Could you check a few things on this drawing? It's one solid part, dimensions in mm from its lowest x, y, z. Give positions to 0.01 mm unless a question says otherwise; leave off trailing zeros. Write each loop counter-clockwise with the first axis right and the second up, starting at its lowest first coordinate (ties: lowest second). Pieces come first, ordered by that corner, then holes. Notation, with made-up numbers: (34, 16) -> (92, 16) arc R19 cw to (92, 27) -> close; hole circle Ø9 at (-4.5, 21.25). An arc over 180 degrees is marked (long way). Use CSV: the item, a comma, the result in double quotes. Start each with the question number.
(1) Suppose I cut it at C-C on y = 2. List the corners of the cut face in (x, z) for me, plus the area to 3 significant figures.
(2) If we mould it in two halves opening along Z, with no side actions, what happens to the marked faces 1, 2 and 3? For each: pulls with the +Z half, pulls with the -Z half, needs draft (parallel to the pull), parting line crosses it, or undercut.
(3) Suppose I cut it at B-B on x = 37.5. List the corners of the cut face in (y, z) for me, plus the area to 3 significant figures.
(4) Suppose I cut it at A-A on z = 37.5. List the corners of the cut face in (x, y) for me.
(5) For pin 1 Ø2 at (x, y) = (62.5, 8.5) entering from +Z (1 decimal); pin 2 Ø4 at (x, y) = (46, 11.5) entering from +Z; pin 3 Ø3 at (x, z) = (51.5, 17.5) entering from -Y, each with a flat end and sliding along its axis, tell me the tip position at first contact or that it passes through.
(6) Suppose I cut it at D-D on z = 5.5. List the corners of the cut face in (x, y) for me, plus the area to 3 significant figures.
(7) I need wall thicknesses on L1, parallel to X at y = 0.75, z = 58.5 (1 decimal); L2, parallel to Z at x = 53, y = 5.75 (1 decimal); L3, parallel to Z at x = 39, y = 9.5. Which ranges of each line are inside material? Lowest first, please. Write a range as [from, to].
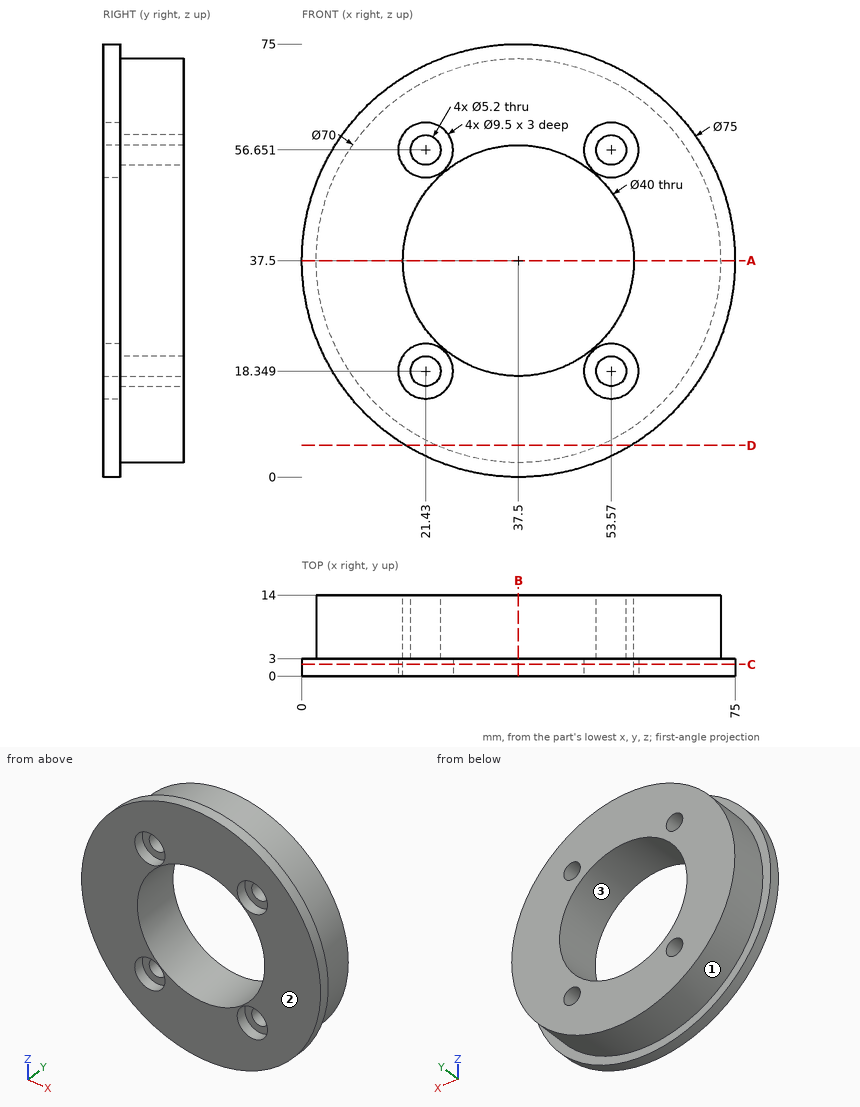
Geometry says:
1,outline,"circle Ø75 at (37.5, 37.5); hole circle Ø9.5 at (21.43, 18.35); hole circle Ø9.5 at (21.43, 56.65); hole circle Ø40 at (37.5, 37.5); hole circle Ø9.5 at (53.57, 18.35); hole circle Ø9.5 at (53.57, 56.65)"
1,area,"2,880 mm²"
2,face 1,"parting line crosses it"
2,face 2,"needs draft"
2,face 3,"undercut"
3,outline,"(0, 0) -> (3, 0) -> (3, 2.5) -> (14, 2.5) -> (14, 17.5) -> (0, 17.5) -> close; (0, 57.5) -> (14, 57.5) -> (14, 72.5) -> (3, 72.5) -> (3, 75) -> (0, 75) -> close"
3,area,"435 mm²"
4,outline,"(0, 0) -> (17.5, 0) -> (17.5, 14) -> (2.5, 14) -> (2.5, 3) -> (0, 3) -> close; (57.5, 0) -> (75, 0) -> (75, 3) -> (72.5, 3) -> (72.5, 14) -> (57.5, 14) -> close"
5,pin 1,"z = 63"
5,pin 2,"z = 71.89"
5,pin 3,"y = 3"
6,outline,"(17.95, 0) -> (57.05, 0) -> (57.05, 3) -> (51.68, 3) -> (51.68, 14) -> (23.32, 14) -> (23.32, 3) -> (17.95, 3) -> close"
6,area,"429 mm²"
7,L1,"[6.4, 17.1], [25.8, 49.2], [57.9, 68.6]"
7,L2,"[6.1, 15.8], [20.9, 24.9], [50.1, 54.1], [59.2, 68.9]"
7,L3,"[2.53, 17.56], [57.44, 72.47]"
